from build123d import *

# Parameters (mm, degrees)
BOSS_EXTRUDE1_DEPTH = 38.1
SKETCH2_R           = 8.1915
CUT_EXTRUDE1_DEPTH  = 3.175
SKETCH3_R           = 8.1915
CUT_EXTRUDE2_DEPTH  = 3.175
SKETCH4_R           = 4.8895
CUT_EXTRUDE3_DEPTH  = 1.6129


with BuildPart() as part:
    # Sketch1 → Boss-Extrude1 (new body)
    with BuildSketch(Plane(origin=(0, 0, 0), x_dir=(1, 0, 0), z_dir=(0, 1, 0))):
        Polygon((0, 0), (0, 38.1), (38.1, 0), align=None)
    extrude(amount=BOSS_EXTRUDE1_DEPTH)

    # Sketch2 → Cut-Extrude1 (cut)
    with BuildSketch(Plane.XY):
        with Locations((19.05, 19.05)):
            Circle(SKETCH2_R)
    extrude(amount=-CUT_EXTRUDE1_DEPTH, mode=Mode.SUBTRACT)

    # Sketch3 → Cut-Extrude2 (cut)
    with BuildSketch(Plane.ZY):
        with Locations((-25.4, 19.05)):
            Circle(SKETCH3_R)
    extrude(amount=-CUT_EXTRUDE2_DEPTH, mode=Mode.SUBTRACT)

    # Sketch4 → Cut-Extrude3 (cut)
    with BuildSketch(Plane.ZY):
        with Locations((-7.62, 19.05)):
            Circle(SKETCH4_R)
    extrude(amount=-CUT_EXTRUDE3_DEPTH, mode=Mode.SUBTRACT)


solid = part.part
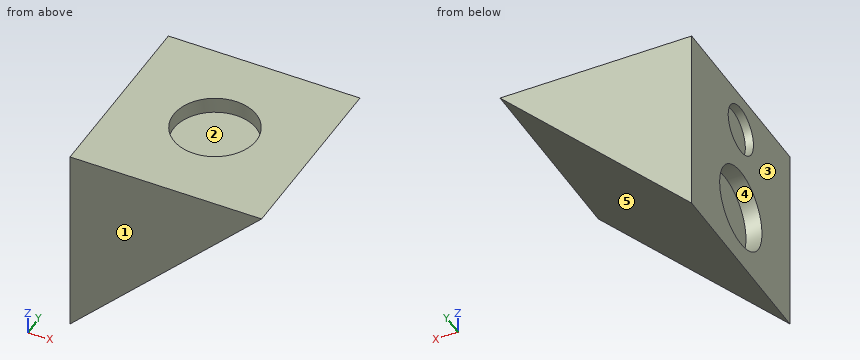
For this review, take the finished solid that the model builds, in its own axes (mm). Face numbers are marked on the shaded views. A direction names the side the tool comes from. Round coordinates to 2 decimals unless told otherwise and drop trailing zeros. Write each loop counter-clockwise with the first axis right and the second up, starting at its lowest first coordinate (ties: lowest second). Pieces come first, ordered by that corner, then holes. Notation, with made-up numbers: (85, 76) - (127, 76) arc R8 ccw to (127, 90) - close; hole circle Ø4 at (47, 77). An arc over 180 degrees is marked (long way). Use a Markdown table: item, result.
Q1. We need section D-D (z = -14). Give the boundary of the cut face in (x, y), plus the area to 3 significant figures.
Derived:
| item | result |
|---|---|
| outline | (0, 0) - (24.1, 0) - (24.1, 38.1) - (0, 38.1) - close |
| area | 918 mm2 |
Q2. We need section C-C (z = -7.62). Give the boundary of the cut face in (x, y), plus the area to 3 significant figures.
Derived:
| item | result |
|---|---|
| outline | (0, 0) - (30.48, 0) - (30.48, 38.1) - (0, 38.1) - (0, 23.94) - (1.61, 23.94) - (1.61, 14.16) - (0, 14.16) - close |
| area | 1,150 mm2 |
Q3. Wall thickness on line 1 along Y through (x, z) = (1.55, -25.4); line 2 along Y through (x, z) = (1.1, -7.62); line 3 along Z through (x, y) = (8, 13): over which ranges is each line inside the solid? List them lowest first.
Derived:
| item | result |
|---|---|
| line 1 | y = 0 to 10.86, 27.24 to 38.1 |
| line 2 | y = 0 to 14.16, 23.94 to 38.1 |
| line 3 | z = -30.1 to 0 |
Q4. We need section B-B (y = 19.05). Give the boundary of the cut face in (x, z) (1 decimal), plus the area to 3 significant figures.
Derived:
| item | result |
|---|---|
| outline | (0, -38.1) - (38.1, 0) - (27.2, 0) - (27.2, -3.2) - (10.9, -3.2) - (10.9, 0) - (0, 0) - (0, -2.7) - (1.6, -2.7) - (1.6, -12.5) - (0, -12.5) - (0, -17.2) - (3.2, -17.2) - (3.2, -33.6) - (0, -33.6) - close |
| area | 606 mm2 |
Q5. Clearance check with flat-ended pins moving along their axes: pin 1 (8 mm diameter, centred on y = 15, z = -9.5, fed in from +X); pin 2 (8 mm diameter, centred on x = 20, y = 16, fed in from +Z) (3 decimals); pin 3 (10 mm diameter, centred on y = 14, z = -33.5, fed in from +X); pin 4 (2 mm diameter, centred on x = 24.5, z = -15.5, fed in from -Y). State where each tip first meets the part, or that it passes through.
Derived:
| item | result |
|---|---|
| pin 1 | stops at x = 32.6 |
| pin 2 | stops at z = -3.175 |
| pin 3 | stops at x = 9.6 |
| pin 4 | passes through |
Q6. Machinability: for the marked faces 4 and 5, which of the approach directions +Z, -Z, +X, -X, +Y, -Y give a long, thin tool a straight path to every point of the face, cutting with its end or side? Answer none if there is none.
Derived:
| item | result |
|---|---|
| face 4 | -X |
| face 5 | -Z, +X, +Y, -Y |
Q7. The part is to be moulded in two halves that separate along X. For the marked faces 1, 2 and 3, say which applies: pulls with the +X half, pulls with the -X half, needs draft (parallel to the pull), parting line crosses it, or undercut.
Derived:
| item | result |
|---|---|
| face 1 | needs draft |
| face 2 | undercut |
| face 3 | pulls with the -X half |
